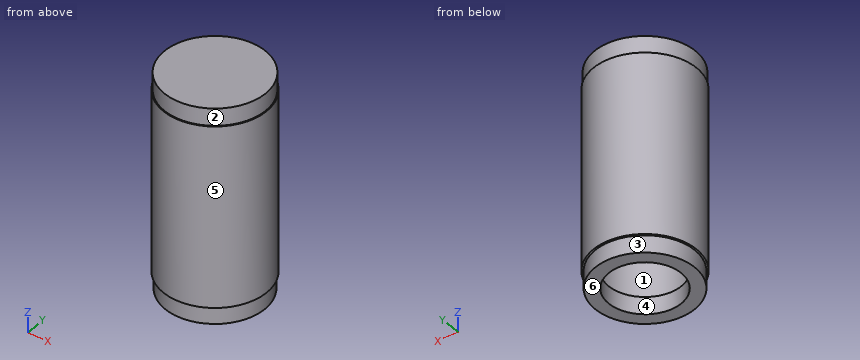
```python
from build123d import *

# Parameters (mm, degrees)
SKETCH1_R           = 30
SKETCH1_R_2         = 25
BOSS_EXTRUDE1_DEPTH = 125
SKETCH2_R           = 25
SKETCH2_R_2         = 21.1
BOSS_EXTRUDE2_DEPTH = 10
SKETCH3_R           = 25
BOSS_EXTRUDE3_DEPTH = 10
SKETCH11_R          = 30
SKETCH11_R_2        = 28.945980101
CUT_EXTRUDE2_DEPTH  = 10
SKETCH12_R          = 30
SKETCH12_R_2        = 29.420954363
CUT_EXTRUDE3_DEPTH  = 10


with BuildPart() as part:
    # Sketch1 → Boss-Extrude1 (new body)
    with BuildSketch(Plane.XY):
        Circle(SKETCH1_R)
        Circle(SKETCH1_R_2, mode=Mode.SUBTRACT)
    extrude(amount=BOSS_EXTRUDE1_DEPTH)

    # Sketch2 → Boss-Extrude2 (add)
    with BuildSketch(Plane.XY):
        Circle(SKETCH2_R)
        Circle(SKETCH2_R_2, mode=Mode.SUBTRACT)
    extrude(amount=BOSS_EXTRUDE2_DEPTH)

    # Sketch3 → Boss-Extrude3 (add)
    with BuildSketch(Plane.XY.offset(115)):
        Circle(SKETCH3_R)
    extrude(amount=BOSS_EXTRUDE3_DEPTH)

    # Sketch11 → Cut-Extrude2 (cut)
    with BuildSketch(Plane(origin=(0, 0, 0), x_dir=(-1, 0, 0), z_dir=(0, 0, -1))):
        Circle(SKETCH11_R)
        Circle(SKETCH11_R_2, mode=Mode.SUBTRACT)
    extrude(amount=-CUT_EXTRUDE2_DEPTH, mode=Mode.SUBTRACT)

    # Sketch12 → Cut-Extrude3 (cut)
    with BuildSketch(Plane.XY.offset(125)):
        Circle(SKETCH12_R)
        Circle(SKETCH12_R_2, mode=Mode.SUBTRACT)
    extrude(amount=-CUT_EXTRUDE3_DEPTH, mode=Mode.SUBTRACT)


solid = part.part
```
Check sheet for the modelled part. Datum: model origin and axes. Units: mm. Face numbers are marked on the shaded views. A direction names the side the tool comes from. Round coordinates to 2 decimals unless told otherwise and drop trailing zeros. Order: outer loops, then holes, each group sorted by start corner. A loop starts at its lowest first (then second) coordinate and runs counter-clockwise, first axis right, second up.
1) Section check A-A (y = 0). Record the boundary of the cut face in (x, z), and give its area (3 significant figures).
2) Section check C-C (z = 106). Record the boundary of the cut face in (x, y).
3) Tool access check on the marked faces 1, 2 and 3. Record the directions out of +Z, -Z, +X, -X, +Y, -Y that give a thin tool (end or side, any length) a straight path to the whole face; none if there is none.
4) Mould release check, pull along X, two halves, no side actions. Record for the marked faces 4, 5 and 6: +X half, -X half, draft (parallel to the pull), parting line (faces both ways), or undercut.
5) Scan lines: line 1 (Y direction, x = 0, z = 3); line 2 (Z direction, x = 24, y = -1.5); line 3 (Y direction, x = 0, z = 83). Record each from-to range of solid material in increasing order.
6) Go/stop test with flat-tipped pins: pin 1 Ø12 at (y, z) = (19, 68.5) entering from +X; pin 2 Ø10 at (x, z) = (-5.5, 16) entering from -Y; pin 3 Ø5 at (y, z) = (10, 70) entering from -X. Record where each tip stops, or that it passes through.
Result:
1. outline: (-30, 10) - (-28.95, 10) - (-28.95, 0) - (-21.1, 0) - (-21.1, 10) - (-25, 10) - (-25, 115) - (25, 115) - (25, 10) - (21.1, 10) - (21.1, 0) - (28.95, 0) - (28.95, 10) - (30, 10) - (30, 115) - (29.42, 115) - (29.42, 125) - (-29.42, 125) - (-29.42, 115) - (-30, 115) - close
1. area: 1,800 mm2
2. outline: circle Ø60 at (0, 0); hole circle Ø50 at (0, 0)
3. face 1: none
3. face 2: +Z
3. face 3: -Z
4. face 4: undercut
4. face 5: parting line
4. face 6: draft
5. line 1: y = -28.95 to -21.1, 21.1 to 28.95
5. line 2: z = 0 to 10, 115 to 125
5. line 3: y = -30 to -25, 25 to 30
6. pin 1: stops at x = 27.04
6. pin 2: stops at y = -30
6. pin 3: stops at x = -29.05
